```python
from build123d import *

# Parameters (mm, degrees)
SKETCH_1_W             = 4
SKETCH_1_H             = 8
SKETCH_1_R             = 0.75
SKETCH_1_W_2           = 1.1
SKETCH_1_H_2           = 1.9
EXTRUDE_1_DEPTH        = 0.7
PATTERN_LINEAR_2_COUNT = 10
PATTERN_LINEAR_2_PITCH = 4


with BuildPart() as part:
    # 草图1 → 凸台-拉伸1 (new body)
    with BuildSketch(Plane(origin=(0, 0, 0), x_dir=(1, 0, 0), z_dir=(0, 1, 0))):
        with Locations((0, 4)):
            Rectangle(SKETCH_1_W, SKETCH_1_H)
        with Locations(Location((0, 6.25, 0), (0, 0, 270))):
            Circle(SKETCH_1_R, mode=Mode.SUBTRACT)
        with Locations((0, 2.75)):
            Rectangle(SKETCH_1_W_2, SKETCH_1_H_2, mode=Mode.SUBTRACT)
    extrude_1 = extrude(amount=EXTRUDE_1_DEPTH)

    # 阵列(线性)2: 凸台-拉伸1 ×10
    with Locations(*[(i * PATTERN_LINEAR_2_PITCH, 0, 0) for i in range(1, PATTERN_LINEAR_2_COUNT)]):
        add(extrude_1)


solid = part.part
```
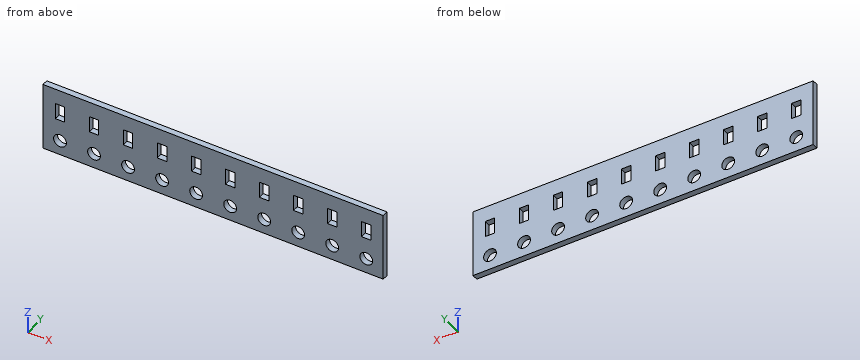
The listing builds one solid part. Answer for the finished solid, in the listing's coordinates (mm). Coordinates: 2 decimals unless noted, no trailing zeros. Loops run counter-clockwise (first coordinate to the right, second up) from the corner with the lowest first, then second, coordinate; pieces in that order, holes last. Notation, with made-up numbers: (81.25, -14.75) -> (129.25, -14.75) arc R33 ccw to (129.25, 24.25) -> close; hole circle Ø5 at (-28.75, 23). An arc over 180 degrees is marked (long way). Use one line per item in the form item = value. Start each with the question number.
Item 1: The part is cut by section B-B on z = -2.75. Count the separate pieces of the cut face and the enclosed holes in it, then the cut area to 3 significant figures.
Item 2: Consider L1, parallel to Z at x = 32, y = 0.45; L2, parallel to Z at x = 27.5, y = 0.6. Determine where each line is inside the solid, lowest interval first. Write a range as [from, to].
Item 3: The part is cut by section A-A on x = 16. Determine the outline of the cut face in (y, z), then the cut area to 3 significant figures.
Answer key:
q1.separate_pieces = 11
q1.enclosed_holes = 0
q1.area = 20.3 mm2
q2.L1 = [-8, -7], [-5.5, -3.7], [-1.8, 0]
q2.L2 = [-8, -6.81], [-5.69, -3.7], [-1.8, 0]
q3.outline = (0, -8) -> (0.7, -8) -> (0.7, -7) -> (0, -7) -> close; (0, -5.5) -> (0.7, -5.5) -> (0.7, -3.7) -> (0, -3.7) -> close; (0, -1.8) -> (0.7, -1.8) -> (0.7, 0) -> (0, 0) -> close
q3.area = 3.22 mm2
